```python
from build123d import *


with BuildPart() as f2:
    # F0 (on Top) → F2 (revolve)
    with BuildSketch(Plane.XY):
        Polygon((19.49287, 0), (20.401696, 1.742762), (23.705291, 1.742762), (25.598362, 2.485143), (20.847125, 2.485143), (22.628838, 5.900095), (32.131314, 5.900095), (33.690315, 7.162142), (23.222743, 7.162142), (24.559028, 10.317261), (36.437124, 10.317261), (37.179504, 11.50507), (25.001479, 11.50507), (25.419937, 12.806245), (37.615031, 12.806245), (37.943818, 13.762723), (25.599279, 13.762723), (25.957957, 15.25722), (25.957957, 15.914798), (38.272608, 15.914798), (38.272608, 16.871275), (26.077516, 16.871275), (26.077516, 18.86609), (38.089752, 18.86609), (37.901918, 19.898646), (25.983186, 19.898646), (25.742499, 21.441443), (37.391759, 21.441443), (37.082178, 22.230875), (25.453674, 22.230875), (24.765017, 23.986951), (35.65881, 23.776108), (34.744199, 24.570378), (24.322445, 24.835132), (23.705291, 25.894463), (33.284654, 25.709061), (32.160349, 26.394593), (23.231866, 26.567398), (22.438888, 27.546959), (30.225785, 27.396249), (28.929776, 28.017683), (22.047411, 28.150887), (21.235704, 28.922867), (27.353505, 28.673161), (25.543135, 29.453492), (20.56286, 29.549882), (19.530335, 30.45997), (23.705291, 30.289564), (22.745302, 30.803315), (19.030804, 30.875207), (17.782392, 31.583648), (21.621624, 31.583648), (20.847125, 32.254733), (16.532759, 32.338235), (15.503824, 33.269163), (20.107782, 33.269163), (19.719002, 34.260551), (14.920684, 34.260551), (14.417998, 35.251565), (19.545402, 35.251565), (19.545402, 36.005594), (14.173682, 36.005594), (13.908926, 37.398864), (19.49287, 37.398864), (19.757625, 38.506024), (13.884857, 38.506024), (13.908926, 39.749626), (19.912066, 39.749626), (20.107782, 40.81), (14.0809, 40.81), (14.307109, 42.041585), (20.414753, 42.041585), (20.728931, 43.273166), (14.64579, 43.273166), (15.247508, 45.147993), (21.168413, 45.147993), (21.596163, 46.773442), (15.503824, 46.773442), (10.511392, 46.977215), (10.511392, 1.742762), (0, 1.946203), (0, 0), align=None)
    revolve(axis=Axis((0, 27.407939, 0), (0, 1, 0)))


solid = f2.part
```
Source: CAD feature listing. Evaluate the final solid. Frame: model axes, mm. A direction names the side the tool comes from. Round coordinates to 2 decimals unless told otherwise and drop trailing zeros. Answer as a JSON object with one key per item and string values. Group by question number.
(1) Ray query, line 1 (Y direction, x = 29, z = 19); line 2 (Z direction, x = 0, y = 16.5); line 3 (Y direction, x = -18.5, z = 16). Return the intervals inside material, ascending. Write a range as [from, to].
(2) Mould query, pull axis Z, two halves, no side actions, for faces 3 (the conical face through (-5.516, 23.974, 24.841)), 4 (the flat face through (-9, 22.231, 24)), 5 (the cylindrical face through (18.643, 35.634, -5.871)), 6 (the conical face through (21.867, 27.538, -6.886)). Classes: +Z half, -Z half, draft (parallel to the pull), parting line (faces both ways), or undercut.
(3) Reachability of faces 1 (the conical face through (-2.914, 28.144, -22.191)), 2 (the conical face through (-0.111, 1.936, 0.498)) from +Z, -Z, +X, -X, +Y, -Y: full face, straight path, thin tool, end or side. Return the list, or none.
(4) First-contact query: pin 1 (12 mm diameter, centred on x = 23.5, z = -11, fed in from +Y); pin 2 (1 mm diameter, centred on y = 5.5, z = -11, fed in from +X); pin 3 (3 mm diameter, centred on y = 25, z = -9.5, fed in from -X). Flat tips, straight axial feed; report the tip coordinate or a pass-through.
Computed values:
{
 "1": {"line 1": "[10.32, 11.51], [12.81, 13.76], [15.91, 16.87], [18.87, 19.9], [21.44, 22.23], [23.8, 24.57]", "line 2": "[-38.27, -10.51], [10.51, 38.27]", "line 3": "[2.04, 2.49], [5.9, 7.16], [10.08, 24.83], [25.88, 26.54], [27.51, 28.1], [28.79, 29.47]"},
 "2": {"face 3": "undercut", "face 4": "draft", "face 5": "parting line", "face 6": "undercut"},
 "3": {"face 1": "none", "face 2": "+Y"},
 "4": {"pin 1": "y = 46.77", "pin 2": "x = 30.35", "pin 3": "x = -34.6"}
}
